Could you check a few things on this model? Use its own coordinates, in mm. Face numbers are marked on the shaded views. A direction names the side the tool comes from. Give positions to 0.01 mm unless a question says otherwise; leave off trailing zeros. Loops run counter-clockwise (first coordinate to the right, second up) from the corner with the lowest first, then second, coordinate; pieces in that order, holes last.
1. I need wall thicknesses on line 1 along Y through (x, z) = (0, 3.75); line 2 along Y through (x, z) = (-2.25, 10.5); line 3 along Y through (x, z) = (4.5, 12.75). Which ranges of each line are inside material? Lowest first, please.
2. Imagine slicing it at B-B (z = 8). List the corners of the cut face in (x, y) for me.
3. Imagine slicing it at C-C (y = -2). List the corners of the cut face in (x, z) for me, plus the area to 3 significant figures.
4. Thinking about a two-plate mould opening in Z: for the marked faces 3, 4 and 5, which applies, +Z half, -Z half, draft (parallel to the pull), parting line (faces both ways), or undercut?
5. Imagine slicing it at A-A (x = 1.5). List the corners of the cut face in (y, z) for me, plus the area to 3 significant figures.
6. Imagine slicing it at D-D (x = -5.5). List the corners of the cut face in (y, z) for me, plus the area to 3 significant figures.
7. For the marked faces 1 and 2, which set-ups out of +Z, -Z, +X, -X, +Y, -Y let a thin tool reach every point of the face, with its end or its side?
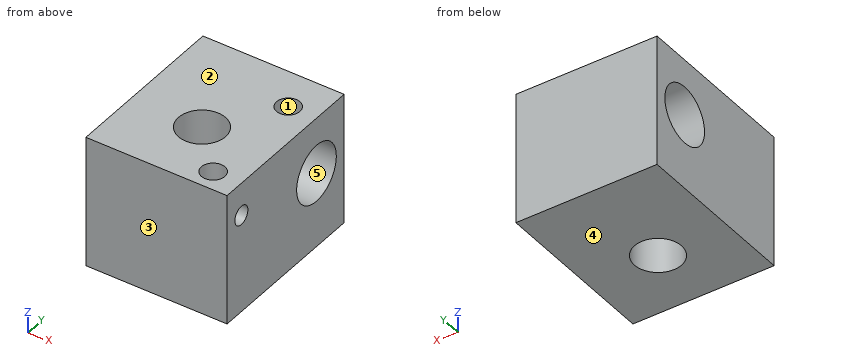
```python
from build123d import *

# Parameters (mm, degrees)
SKETCH1_W                           = 15
SKETCH1_H                           = 18
BOSS_EXTRUDE1_DEPTH                 = 14
SKETCH2_R                           = 2.5
CUT_EXTRUDE1_DEPTH                  = 15
SKETCH3_R                           = 3.05
CUT_EXTRUDE2_DEPTH                  = 16
TALADRO_ROSCADO_M31_D               = 2.5
TALADRO_ROSCADO_M31_DEPTH           = 4
TALADRO_ROSCADO_M31_TIP             = 0.751075774
DI_METRO_DE_TALADRO_2_8_2_8_1_D     = 2
DI_METRO_DE_TALADRO_2_8_2_8_1_DEPTH = 12
DI_METRO_DE_TALADRO_2_8_2_8_1_TIP   = 0.600860619


with BuildPart() as part:
    # Sketch1 → Boss-Extrude1 (new body)
    with BuildSketch(Plane.XY):
        Rectangle(SKETCH1_W, SKETCH1_H)
    extrude(amount=BOSS_EXTRUDE1_DEPTH)

    # Sketch2 → Cut-Extrude1 (cut, through all)
    with BuildSketch(Plane(origin=(0, 0, 0), x_dir=(-1, 0, 0), z_dir=(0, 0, -1))):
        with Locations((0, -2)):
            Circle(SKETCH2_R)
    extrude(amount=-CUT_EXTRUDE1_DEPTH, mode=Mode.SUBTRACT)

    # Sketch3 → Cut-Extrude2 (cut, through all)
    with BuildSketch(Plane(origin=(7.5, 0, 0), x_dir=(0, 0, -1), z_dir=(1, 0, 0))):
        with Locations((-8, 4.75)):
            Circle(SKETCH3_R)
    extrude(amount=-CUT_EXTRUDE2_DEPTH, mode=Mode.SUBTRACT)

    # Taladro roscado M31
    with Locations(Plane(origin=(-2.648652683, -2.97524228, 14), x_dir=(1, 0, 0), z_dir=(0, 0, 1))):
        with Locations((7.148652683, 7.72524228), (7.148652683, -3.82475772)):
            Hole(TALADRO_ROSCADO_M31_D / 2, depth=TALADRO_ROSCADO_M31_DEPTH)
            with Locations((0, 0, -(TALADRO_ROSCADO_M31_DEPTH + TALADRO_ROSCADO_M31_TIP / 2))):  # 118° drill point
                Cone(0, TALADRO_ROSCADO_M31_D / 2, TALADRO_ROSCADO_M31_TIP, mode=Mode.SUBTRACT)

    # Diámetro de taladro Ø2.8 (2.8)1
    with Locations(Plane(origin=(7.5, -6.8, 10.5), x_dir=(0, 0, 1), z_dir=(1, 0, 0))):
        with Locations((0, 0)):
            Hole(DI_METRO_DE_TALADRO_2_8_2_8_1_D / 2, depth=DI_METRO_DE_TALADRO_2_8_2_8_1_DEPTH)
            with Locations((0, 0, -(DI_METRO_DE_TALADRO_2_8_2_8_1_DEPTH + DI_METRO_DE_TALADRO_2_8_2_8_1_TIP / 2))):  # 118° drill point
                Cone(0, DI_METRO_DE_TALADRO_2_8_2_8_1_D / 2, DI_METRO_DE_TALADRO_2_8_2_8_1_TIP, mode=Mode.SUBTRACT)


solid = part.part
```
Derived:
1. line 1: y = -9 to -4.5, 0.5 to 9
1. line 2: y = -9 to -7.8, -5.8 to -3.09, -0.91 to 3, 6.5 to 9
1. line 3: y = -9 to -8.05, -5.55 to 3.5, 6 to 9
2. outline: (-7.5, -9) - (7.5, -9) - (7.5, 1.7) - (-7.5, 1.7) - close; (-7.5, 7.8) - (7.5, 7.8) - (7.5, 9) - (-7.5, 9) - close; hole circle Ø5 at (0, -2)
3. outline: (-7.5, 0) - (-2.5, 0) - (-2.5, 14) - (-7.5, 14) - close; (2.5, 0) - (7.5, 0) - (7.5, 14) - (2.5, 14) - close
3. area: 140 mm2
4. face 3: draft
4. face 4: -Z half
4. face 5: undercut
5. outline: (-9, 0) - (-4, 0) - (-4, 14) - (-9, 14) - close; (0, 0) - (9, 0) - (9, 14) - (0, 14) - close; hole circle Ø2 at (-6.8, 10.5); hole circle Ø6.1 at (4.75, 8)
5. area: 164 mm2
6. outline: (-9, 0) - (9, 0) - (9, 14) - (-9, 14) - close; hole circle Ø6.1 at (4.75, 8)
6. area: 223 mm2
7. face 1: +Z
7. face 2: +Z, +X, -X, +Y, -Y
